Can you work these out from the model? Positions are in its coordinate system, mm. A direction names the side the tool comes from. Give positions to 0.01 mm unless a question says otherwise; leave off trailing zeros. Order: outer loops, then holes, each group sorted by start corner. A loop starts at its lowest first (then second) coordinate and runs counter-clockwise, first axis right, second up. Notation, with made-up numbers: (17, 62.5) - (41, 62.5) arc R26 ccw to (41, 89.5) - close; hole circle Ø2 at (60.5, -17). An arc over 180 degrees is marked (long way). Answer as a JSON object with one key per item and string values.
```python
from build123d import *
from build123d.topology import SkipClean

# Parameters (mm, degrees)
CUT_SWEEP1_PITCH = 1.27


with BuildPart() as part:
    # Sketch1 → Revolve1 (revolve)
    with BuildSketch(Plane.XY, mode=Mode.PRIVATE) as revolve1_sk:
        Polygon((-12.3063, 6.3754), (-12.3063, 5.6007), (-7.772716776, 2.1844), (12.3063, 2.1844), (12.3063, 2.51206), (12.3063, 5.55625), (8.266523424, 5.55625), (-1.6637, 5.55625), (-1.6637, 5.4864), (-7.9375, 5.4864), (-7.9375, 6.3754), align=None)
    revolve(revolve1_sk.sketch.rotate(Axis((-12.3063, 0, 0), (1, 0, 0)), 90), axis=Axis((-12.3063, 0, 0), (1, 0, 0)))

    # Cut-Sweep1: the profile of Sketch4 profile screwed along a right-hand helix of 11 turns, 8 arcs to a turn; built about Z, then put on its axis
    cut_sweep1_z = Axis((0, 0, 0), (0, 0, 1))
    cut_sweep1_corners = [(5.55655, 0, 0.000173205), (5.55655, 0, -1.111423205), (4.731360803, 0, -0.635), (4.731360803, 0, -0.47625)]
    with BuildLine(mode=Mode.PRIVATE) as cut_sweep1_profile:
        Line(cut_sweep1_corners[0], cut_sweep1_corners[1])
        Line(cut_sweep1_corners[1], cut_sweep1_corners[2])
        Line(cut_sweep1_corners[2], cut_sweep1_corners[3])
        Line(cut_sweep1_corners[3], cut_sweep1_corners[0])
    cut_sweep1_cap = Face(cut_sweep1_profile.wire())
    cut_sweep1_turn_angles = [0, 22.5, 45, 67.5, 90, 112.5, 135, 157.5, 180, 202.5, 225, 247.5, 270, 292.5, 315, 337.5, 360]
    cut_sweep1_turn_weights = [1, 0.9238795325112867, 1, 0.9238795325112867, 1, 0.9238795325112867, 1, 0.9238795325112867, 1, 0.9238795325112867, 1, 0.9238795325112867, 1, 0.9238795325112867, 1, 0.9238795325112867, 1]
    cut_sweep1_turn_rails = [Edge.make_bspline([Vector(p[0], p[1], 0).rotate(cut_sweep1_z, cut_sweep1_turn_angles[k]) / cut_sweep1_turn_weights[k] + Vector(0, 0, p[2] + CUT_SWEEP1_PITCH * cut_sweep1_turn_angles[k] / 360) for k in range(17)], [0, 0, 0, 1, 1, 2, 2, 3, 3, 4, 4, 5, 5, 6, 6, 7, 7, 8, 8, 8], 2, cut_sweep1_turn_weights) for p in cut_sweep1_corners]
    cut_sweep1_turn_sides = [Face.make_surface_from_curves(cut_sweep1_turn_rails[p[0]], cut_sweep1_turn_rails[p[1]]) for p in [(0, 1), (1, 2), (2, 3), (3, 0)]]
    cut_sweep1_turn = Solid(Shell([*cut_sweep1_turn_sides, cut_sweep1_cap, cut_sweep1_cap.rotate(cut_sweep1_z, 360).moved(Location((0, 0, CUT_SWEEP1_PITCH * 360 / 360)))]))
    cut_sweep1_each = [*[cut_sweep1_turn.moved(Location((0, 0, CUT_SWEEP1_PITCH * i))) for i in range(11)]]
    add(Plane(origin=(12.3063, 0, 0), x_dir=(0, 1, 0), z_dir=(-1, 0, 0)) * Compound([cut_sweep1_each[i] for i in range(0, 11, 2)]), mode=Mode.SUBTRACT)
    add(Plane(origin=(12.3063, 0, 0), x_dir=(0, 1, 0), z_dir=(-1, 0, 0)) * Compound([cut_sweep1_each[i] for i in range(1, 11, 2)]), mode=Mode.SUBTRACT)

    # Sketch5 → Cut-Revolve1 (revolve, cut)
    with BuildSketch(Plane.XY, mode=Mode.PRIVATE) as cut_revolve1_sk:
        Polygon((12.3063, 2.51206), (9.428602239, 4.680560803), (8.158602239, 4.680560803), (7.282913042, 5.55625), (12.3063, 5.55625), align=None)
        Polygon((-1.6637, 5.55625), (-1.6637, 4.680560803), (-0.3937, 4.680560803), (0.481989197, 5.55625), align=None)
    revolve(cut_revolve1_sk.sketch.rotate(Axis((0, 0, 0), (-1, 0, 0)), 90), axis=Axis((0, 0, 0), (-1, 0, 0)), mode=Mode.SUBTRACT)

    # Sketch6 → Revolve2 (revolve)
    with SkipClean():  # the faces are left unmerged after this step: merging them gives an invalid solid
        with BuildSketch(Plane.XY, mode=Mode.PRIVATE) as revolve2_sk:
            Polygon((-0.3937, 4.680560803), (8.158602239, 4.680560803), (7.282913042, 5.55625), (0.481989197, 5.55625), align=None)
        revolve(revolve2_sk.sketch.rotate(Axis((0, 0, 0), (-1, 0, 0)), 90), axis=Axis((0, 0, 0), (-1, 0, 0)))
    add(part.part.scale(1), mode=Mode.REPLACE)  # the faces are merged on a copy


solid = part.part
```
Q1. If we section it at B-B, the plane x = -10: Please give me the cut outline in (y, z), then the cut area to 3 significant figures.
Recorded:
{"outline": "circle Ø12.75 at (0, 0); hole circle Ø7.73 at (0, 0)", "area": "80.8 mm^2"}
Q2. I need wall thicknesses on L1, parallel to Y at x = 4.75, z = 0; L2, parallel to X at y = 5, z = 1.5; L3, parallel to Y at x = -9, z = -0.5. Which ranges of each line are inside material? Lowest first, please.
Recorded:
{"L1": "y = -5.56 to -2.18, 2.18 to 5.56", "L2": "x = -11.8 to -1.66, 0.15 to 7.62", "L3": "y = -6.36 to -3.07, 3.07 to 6.36"}
Q3. We'd pull the mould along Z, two halves only. Please class faces 3 (the face through (8.785, -1.406, -4.464)), 4 (the face through (-7.938, -5, -3)), 5 (the face through (-8, 2.3, -0.5)): released by +Z, released by -Z, zero draft, split by the parting line, or undercut.
Recorded:
{"face 3": "split by the parting line", "face 4": "zero draft", "face 5": "undercut"}
Q4. I'm going to push flat-ended pins straight in: pin 1 Ø2 at (x, y) = (2, 2) entering from -Z; pin 2 Ø1 at (y, z) = (-5, -0.5) entering from -X; pin 3 Ø2 at (x, y) = (-5, 5) entering from -Z. Where does each tip first touch, or does it pass through?
Recorded:
{"pin 1": "stops at z = -5.47", "pin 2": "stops at x = -12.21", "pin 3": "stops at z = -3.76"}
Q5. Which directions (+Z, -Z, +X, -X, +Y, -Y) give clear straight access to the entire face, cutting with the end or side of a thin tool? Please do faces 1 (the face through (-4.84, -0.24, -5.48)), 2 (the face through (12.13, 1.61, 2.1)).
Recorded:
{"face 1": "none", "face 2": "+X"}
